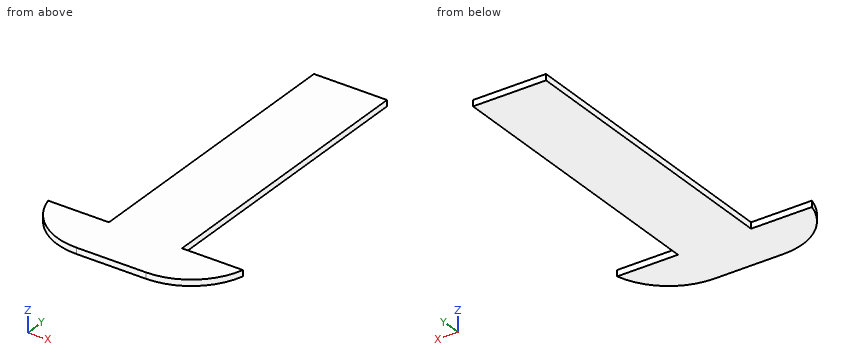
```python
from build123d import *

# Parameters (mm, degrees)
F1_DEPTH    = 3.175
F2_T1_DEPTH = 166.5877767412


# Not quite as in the source:
# - a fillet or chamfer that OpenCascade refuses, or shapes differently, is made with other operations: its cross-section is extruded or revolved along the edge and cut away or added


with BuildPart() as f1:
    # F0 (on Top) → F1 (new body)
    with BuildSketch(Plane.XY):
        Polygon((19.05, -76.2), (19.05, 76.2), (-19.05, 76.2), (-19.05, -76.2), (-50.8, -76.2), (-50.8, -101.6), (50.8, -101.6), (50.8, -76.2), align=None)
    extrude(amount=F1_DEPTH)

    # F2: fillet of radius 33.7265634664 on 2 edges, made by hand

    # F2_s2 → F2_t1 (cut)
    with BuildSketch(Plane.XY.offset(-81.7063883706)):
        with BuildLine():
            ThreePointArc((-50.8, -76.2), (-38.8135156804, -94.5033769622), (-18.1174446518, -101.6))
            Line((-18.1174446518, -101.6), (-50.8, -101.6))
            Line((-50.8, -101.6), (-50.8, -76.2))
        make_face()
        with BuildLine():
            ThreePointArc((18.1174446518, -101.6), (38.8135156804, -94.5033769622), (50.8, -76.2))
            Line((50.8, -76.2), (50.8, -101.6))
            Line((50.8, -101.6), (18.1174446518, -101.6))
        make_face()
    extrude(amount=F2_T1_DEPTH, mode=Mode.SUBTRACT)


solid = f1.part
```
Verification items for the finished model (mm, model axes). Coordinates: 2 decimals unless noted, no trailing zeros. Loops run counter-clockwise (first coordinate to the right, second up) from the corner with the lowest first, then second, coordinate; pieces in that order, holes last. Notation, with made-up numbers: (88.25, 29.25) - (143.25, 29.25) arc R30 ccw to (143.25, 61.25) - close; hole circle Ø2 at (66.5, 73.5). An arc over 180 degrees is marked (long way). Return JSON: item names as keys, results as strings.
1. Section check A-A, the plane z = 0.75. Record the boundary of the cut face in (x, y), then the cut area to 3 significant figures.
Established:
{"outline": "(-50.8, -76.2) arc R33.73 ccw to (-18.12, -101.6) - (18.12, -101.6) arc R33.73 ccw to (50.8, -76.2) - (19.05, -76.2) - (19.05, 76.2) - (-19.05, 76.2) - (-19.05, -76.2) - close", "area": "7,960 mm2"}
2. Go/stop test with flat-tipped pins: pin 1 (1 mm diameter, centred on x = -27.5, z = 1.5, fed in from +Y); pin 2 (1 mm diameter, centred on y = -9, z = 2, fed in from -X). Record where each tip stops, or that it passes through.
Established:
{"pin 1": "stops at y = -76.2", "pin 2": "stops at x = -19.05"}
3. Section check B-B, the plane y = -5. Record the boundary of the cut face in (x, z) (3 decimals), then the cut area to 3 significant figures.
Established:
{"outline": "(-19.05, 0) - (19.05, 0) - (19.05, 3.175) - (-19.05, 3.175) - close", "area": "121 mm2"}
4. Section check C-C, the plane x = 22. Record the boundary of the cut face in (y, z) (3 decimals), then the cut area to 3 significant figures.
Established:
{"outline": "(-101.376, 0) - (-76.2, 0) - (-76.2, 3.175) - (-101.376, 3.175) - close", "area": "79.9 mm2"}
5. Thickness scan on L1, parallel to X at y = -62, z = 0.55; L2, parallel to Y at x = 37, z = 0.55; L3, parallel to X at y = -82.5, z = 1.85. Record the ranges inside material, lowest first.
Established:
{"L1": "x = -19.05 to 19.05", "L2": "y = -95.82 to -76.2", "L3": "x = -48.51 to 48.51"}
